Study the drawing (mm; zero at the part's minimum x, y, z) and answer. Round coordinates to 2 decimals unless told otherwise and drop trailing zeros. Order: outer loops, then holes, each group sorted by start corner. A loop starts at its lowest first (then second) coordinate and runs counter-clockwise, first axis right, second up. Notation, with made-up numbers: (-14.5, 55) - (19.5, 55) arc R22 ccw to (19.5, 74) - close; hole circle Ø10 at (-8, 15.5). An arc over 180 degrees is marked (long way). Put each result on its own line as item: value. Start each with the question number.
Q1. Each of these flat-tipped pins is pushed along its axis until it touches: pin 1 Ø6 at (x, y) = (53, 34.5) entering from +Z; pin 2 Ø6 at (x, y) = (52.5, 53) entering from +Z; pin 3 Ø3 at (x, z) = (12.5, 76) entering from -Y; pin 4 Ø1 at (x, y) = (38.5, 35) entering from +Z. Where does it stop, or does it pass through?
Q2. For a pull along Z with two mould halves and no side action, classify the marked faces 1, 2 and 3 as pulls with the +Z half, pulls with the -Z half, needs draft (parallel to the pull), parting line crosses it, or undercut.
Q3. Find the intervals of material crossed by line 1 along Z through (x, y) = (31.5, 4) (1 decimal); line 2 along Z through (x, y) = (37.5, 45) (1 decimal); line 3 along X through (y, z) = (22, 123) (1 decimal), in increasing order. Write a range as from..to.
Q4. Section C-C on z = 112 is taken. Give the vertices of the cut face in (x, y) (1 decimal), then the cut area to 3 significant figures.
Q5. Section A-A on x = 23.5 is taken. Give the vertices of the cut face in (y, z) (1 decimal).
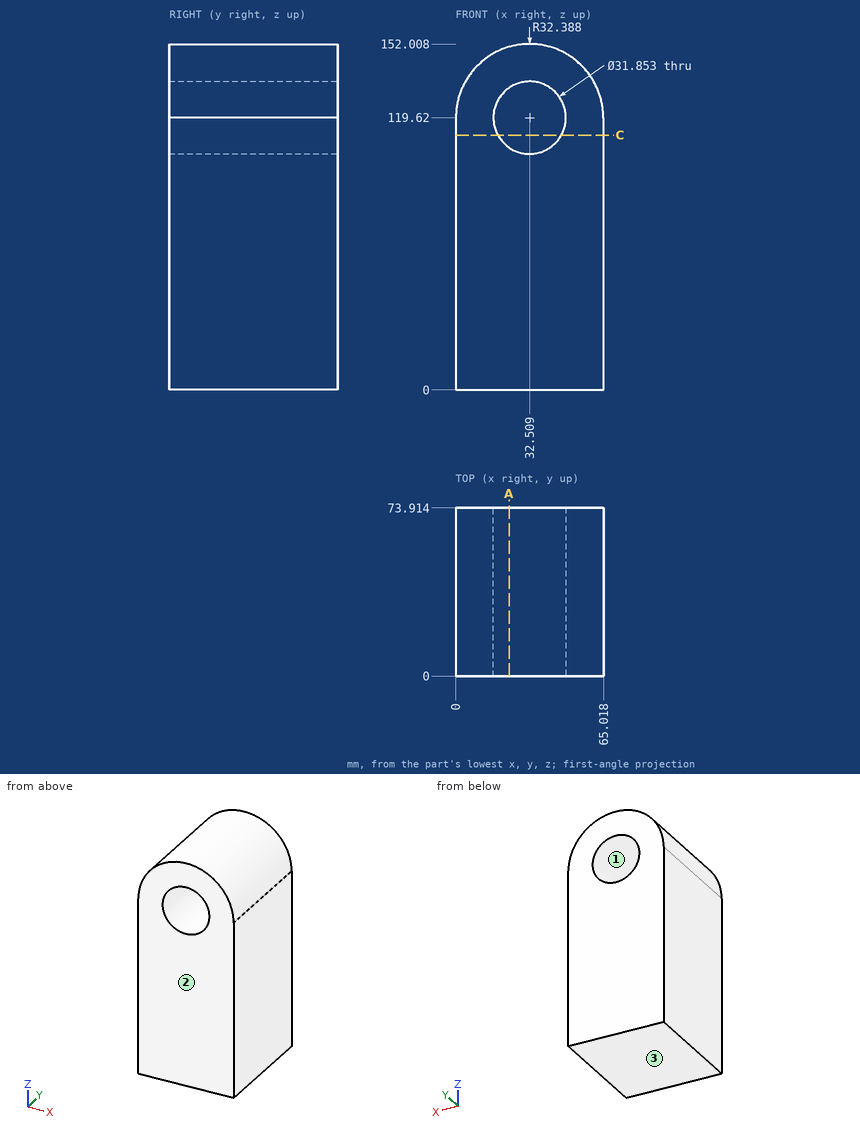
Findings:
1. pin 1: z = 146.88
1. pin 2: z = 147.19
1. pin 3: y = 0
1. pin 4: z = 151.54
2. face 1: undercut
2. face 2: needs draft
2. face 3: pulls with the -Z half
3. line 1: 0..103.7, 135.5..152
3. line 2: 0..104.5, 134.7..151.6
3. line 3: 0.3..16.9, 48.1..64.7
4. outline: (0, 0) - (18.5, 0) - (18.5, 73.9) - (0, 73.9) - close; (46.5, 0) - (65, 0) - (65, 73.9) - (46.5, 73.9) - close
4. area: 2,740 mm2
5. outline: (0, 0) - (73.9, 0) - (73.9, 106.5) - (0, 106.5) - close; (0, 132.8) - (73.9, 132.8) - (73.9, 150.7) - (0, 150.7) - close
